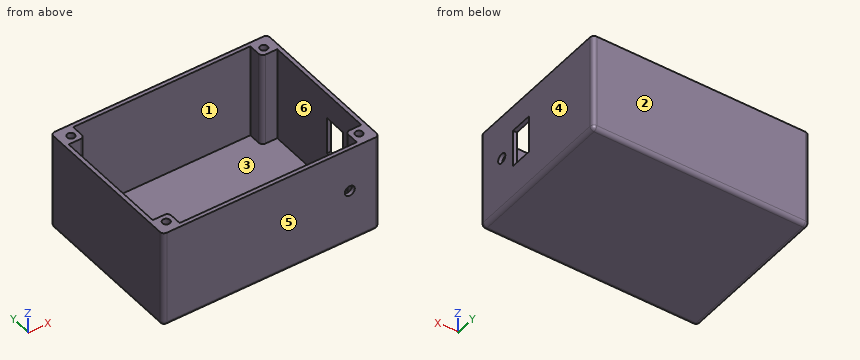
```python
from build123d import *

# Parameters (mm, degrees)
SKETCH_W        = 110
SKETCH_H        = 80
PAD_DEPTH       = 50
SKETCH001_R     = 1.9
POCKET_DEPTH    = 48
FILLET_R        = 2
FILLET001_R     = 2
SKETCH002_R     = 2.55
SKETCH002_W     = 11.5
SKETCH002_H     = 19.1
POCKET001_DEPTH = 5
SKETCH003_R     = 2.55
POCKET002_DEPTH = 5


with BuildPart() as part:
    # Sketch → Pad (new body)
    with BuildSketch(Plane.XY):
        with Locations((55, 40)):
            Rectangle(SKETCH_W, SKETCH_H)
    extrude(amount=PAD_DEPTH)

    # Sketch001 (on Face6 of Pad) → Pocket (cut)
    with BuildSketch(Plane.XY.offset(50)):
        with Locations((6, 74)):
            Circle(SKETCH001_R)
        with Locations((104, 74)):
            Circle(SKETCH001_R)
        with Locations((104, 6)):
            Circle(SKETCH001_R)
        with Locations((6, 6)):
            Circle(SKETCH001_R)
        Polygon((2, 10), (10, 10), (10, 2), (100, 2), (100, 10), (108, 10), (108, 70), (100, 70), (100, 78), (10, 78), (10, 70), (2, 70), align=None)
    extrude(amount=-POCKET_DEPTH, mode=Mode.SUBTRACT)

    # Fillet
    fillet_edges = [part.edges().sort_by_distance(p)[0] for p in [
        (0, 80, 25),
        (0, 40, 0),
        (0, 0, 25),
        (55, 0, 0),
        (110, 0, 25),
        (110, 80, 25),
        (110, 40, 0),
        (55, 80, 0),
    ]]
    fillet(fillet_edges, radius=FILLET_R)

    # Fillet001
    fillet001_edges = [part.edges().sort_by_distance(p)[0] for p in [
        (100, 10, 26),
        (100, 70, 26),
        (10, 70, 26),
        (10, 10, 26),
    ]]
    fillet(fillet001_edges, radius=FILLET001_R)

    # Sketch002 (on Face22 of Fillet001) → Pocket001 (cut)
    with BuildSketch(Plane.YZ.offset(110)):
        with Locations((15, 27.5)):
            Circle(SKETCH002_R)
        with Locations((28.75, 27.5)):
            Rectangle(SKETCH002_W, SKETCH002_H)
    extrude(amount=-POCKET001_DEPTH, mode=Mode.SUBTRACT)

    # Sketch003 (on Face18 of Pocket001) → Pocket002 (cut)
    with BuildSketch(Plane.XZ):
        with Locations((95, 27.5)):
            Circle(SKETCH003_R)
    extrude(amount=-POCKET002_DEPTH, mode=Mode.SUBTRACT)


solid = part.part
```
Work out the finished part from the listing and answer in its coordinate system (mm). Face numbers are marked on the shaded views. A direction names the side the tool comes from. Give positions to 0.01 mm unless a question says otherwise; leave off trailing zeros. Write each loop counter-clockwise with the first axis right and the second up, starting at its lowest first coordinate (ties: lowest second). Pieces come first, ordered by that corner, then holes. Notation, with made-up numbers: (-34.5, 44) -> (17.5, 44) arc R22 cw to (17.5, 59) -> close; hole circle Ø1 at (-16, 59). An arc over 180 degrees is marked (long way). Write each question's results on one line, items separated by ' | '.
1. Find section A-A on y = 15. Determine the outline of the cut face in (x, z), and give its area (3 significant figures).
Data:
outline: (0, 2) arc R2 ccw to (2, 0) -> (108, 0) arc R2 ccw to (110, 2) -> (110, 24.95) -> (108, 24.95) -> (108, 2) -> (2, 2) -> (2, 50) -> (0, 50) -> close; (108, 30.05) -> (110, 30.05) -> (110, 50) -> (108, 50) -> close | area: 400 mm^2
2. Find section D-D on y = 47. Determine the outline of the cut face in (x, z).
Data:
outline: (0, 2) arc R2 ccw to (2, 0) -> (108, 0) arc R2 ccw to (110, 2) -> (110, 50) -> (108, 50) -> (108, 2) -> (2, 2) -> (2, 50) -> (0, 50) -> close
3. Find section C-C on x = 95. Determine the outline of the cut face in (y, z).
Data:
outline: (0, 2) arc R2 ccw to (2, 0) -> (78, 0) arc R2 ccw to (80, 2) -> (80, 50) -> (78, 50) -> (78, 2) -> (2, 2) -> (2, 24.95) -> (0, 24.95) -> close; (0, 30.05) -> (2, 30.05) -> (2, 50) -> (0, 50) -> close
4. Straight lines are drawn through the part: L1, parallel to Y at x = 6, z = 32.5; L2, parallel to X at y = 74, z = 32; L3, parallel to Y at x = 5, z = 17. For each, find the intervals that lie inside material, in ascending order.
Data:
L1: 0 to 4.1, 7.9 to 10, 70 to 72.1, 75.9 to 80 | L2: 0 to 4.1, 7.9 to 10, 100 to 102.1, 105.9 to 110 | L3: 0 to 4.38, 7.62 to 10, 70 to 72.38, 75.62 to 80
5. Determine the mould class of the marked faces 1, 2, 3 and 4 for opening direction Y: +Y half, -Y half, draft (parallel to the pull), parting line (faces both ways), or undercut.
Data:
face 1: undercut | face 2: +Y half | face 3: undercut | face 4: draft
6. A tool of negligible diameter and unlimited length cuts with its end or side. For the marked faces 5 and 6, from which of +Z, -Z, +X, -X, +Y, -Y can it reach the whole face along a straight path? Write none if from no direction.
Data:
face 5: +Z, -Z, +X, -X, -Y | face 6: +Z
7. Each of these flat-tipped pins is pushed along its axis until it touches: pin 1 Ø0.6 at (x, z) = (108.5, 25.5) entering from -Y; pin 2 Ø0.6 at (x, z) = (109, 29.5) entering from +Y; pin 3 Ø0.6 at (x, y) = (109, 26.5) entering from -Z. Where does it stop, or does it pass through?
Data:
pin 1: y = 0.01 | pin 2: y = 79.87 | pin 3: z = 0.13
8. Find section B-B on z = 23. Give the number of separate pieces and of enclosed holes in the cut face, and give its area (3 significant figures).
Data:
separate pieces: 1 | enclosed holes: 4 | area: 925 mm^2
